Autodesk Inventor part; units mm, degrees
ref_plane "YZ Plane" through (0, 0, 0) normal (1, 0, 0) x (0, 1, 0)
ref_plane "XZ Plane" through (0, 0, 0) normal (0, 1, 0) x (-1, 0, 0)
ref_plane "XY Plane" through (0, 0, 0) normal (0, 0, 1) x (1, 0, 0)
sketch "Sketch1" plane through (0, 0, 0) normal (0, 1, 0) x (-1, 0, 0)
  line L0 (17.5, -7.5) -> (-17.5, -7.5)
  line L1 (-17.5, -7.5) -> (-17.5, 7.5)
  line L2 (-17.5, 7.5) -> (17.5, 7.5)
  line L3 (17.5, 7.5) -> (17.5, -7.5)
  line L4 (17.5, -7.5) -> (-17.5, 7.5) construction
  line L5 (-17.5, -7.5) -> (17.5, 7.5) construction
  line L6 (11.75, -6.1) -> (-11.75, -6.1)
  line L7 (-11.75, -6.1) -> (-11.75, 6.1)
  line L8 (-11.75, 6.1) -> (11.75, 6.1)
  line L9 (11.75, 6.1) -> (11.75, -6.1)
  line L10 (11.75, -6.1) -> (-11.75, 6.1) construction
  line L11 (-11.75, -6.1) -> (11.75, 6.1) construction
  circle A0 centre (13.25, 0) radius 0.75
  circle A1 centre (-13.1, 0) radius 0.75
  point P0 (0, 0)
  dimension "d37" = 35
  dimension "d38" = 15
  dimension "d39" = 5.75
  dimension "d40" = 5.75
  dimension "d41" = 12.2
  dimension "d42" = 1.5
  dimension "d43" = 1.5
  dimension "d44" = 4.25
  dimension "d45" = 5.15
extrude "Extrusion4" add sketch "Sketch1" along normal blind 2
properties part number "servo housing lid"
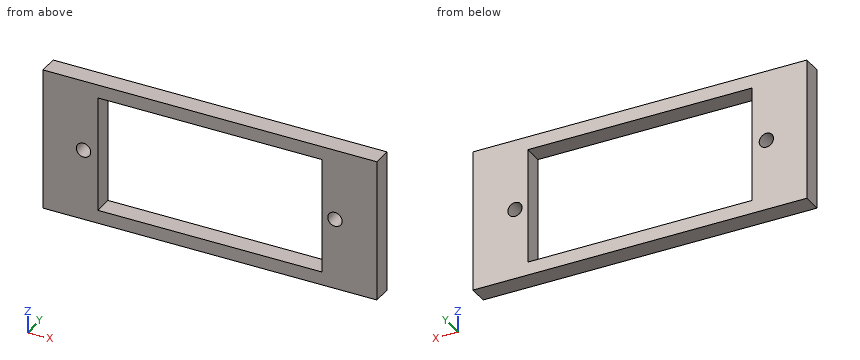
Source: CAD feature listing. Evaluate the final solid. Frame: model axes, mm. Coordinates: 2 decimals unless noted, no trailing zeros. Loops run counter-clockwise (first coordinate to the right, second up) from the corner with the lowest first, then second, coordinate; pieces in that order, holes last. Notation, with made-up numbers: (58, 78) -> (80, 78) arc R16 ccw to (80, 106) -> close; hole circle Ø2 at (78.5, -32). An arc over 180 degrees is marked (long way). One line per item, written item: value. Start each with the question number.
Q1. Line query: line 1 along X through (y, z) = (1.15, -3); line 2 along Z through (x, y) = (-13.25, 0.8); line 3 along Z through (x, y) = (-1, 1.25). Output: solid intervals per line, ascending.
Q2. Section query A-A, the plane x = 6.5. Return the cut outline in (y, z).
Q3. Section query D-D, the plane y = 1.5. Return the cut outline in (x, z), and give its area (3 significant figures).
Q4. Contact query for flat-ended pins moving along their axis: P1, Ø2.5, axis at x = 13.1, z = 0, coming from the -Y side; P2, Ø1.2, axis at x = -13.25, z = 0, coming from the -Y side. Output: stop coordinate, or through.
Q5. Section query B-B, the plane z = 0. Return the cut outline in (x, y), and give its area (3 significant figures).
Q6. Section query C-C, the plane z = 4.25. Return the cut outline in (x, y).
Results:
1. line 1: -17.5 to -11.75, 11.75 to 17.5
1. line 2: -7.5 to -0.75, 0.75 to 7.5
1. line 3: -7.5 to -6.1, 6.1 to 7.5
2. outline: (0, -7.5) -> (2, -7.5) -> (2, -6.1) -> (0, -6.1) -> close; (0, 6.1) -> (2, 6.1) -> (2, 7.5) -> (0, 7.5) -> close
3. outline: (-17.5, -7.5) -> (17.5, -7.5) -> (17.5, 7.5) -> (-17.5, 7.5) -> close; hole circle Ø1.5 at (-13.25, 0); hole (-11.75, -6.1) -> (11.75, -6.1) -> (11.75, 6.1) -> (-11.75, 6.1) -> close; hole circle Ø1.5 at (13.1, 0)
3. area: 235 mm^2
4. P1: y = 0
4. P2: through
5. outline: (-17.5, 0) -> (-14, 0) -> (-14, 2) -> (-17.5, 2) -> close; (-12.5, 0) -> (-11.75, 0) -> (-11.75, 2) -> (-12.5, 2) -> close; (11.75, 0) -> (12.35, 0) -> (12.35, 2) -> (11.75, 2) -> close; (13.85, 0) -> (17.5, 0) -> (17.5, 2) -> (13.85, 2) -> close
5. area: 17.0 mm^2
6. outline: (-17.5, 0) -> (-11.75, 0) -> (-11.75, 2) -> (-17.5, 2) -> close; (11.75, 0) -> (17.5, 0) -> (17.5, 2) -> (11.75, 2) -> close
